```python
from build123d import *

# Parameters (mm, degrees)
BOSS_EXTRUDE1_DEPTH = 8
SKETCH2_R           = 25
BOSS_EXTRUDE2_DEPTH = 1.5
BOSS_EXTRUDE3_START = 1.5
SKETCH3_R           = 25
BOSS_EXTRUDE3_DEPTH = 1.5
SKETCH4_R           = 8
CUT_EXTRUDE1_DEPTH  = 38.027017163
FILLET1_R           = 4


with BuildPart() as part:
    # Sketch1 → Boss-Extrude1 (new body)
    with BuildSketch(Plane(origin=(0, 0, 0), x_dir=(1, 0, 0), z_dir=(0, 1, 0))):
        with BuildLine():
            ThreePointArc((-13.903357517, 20.777310936), (-23.090394822, -9.582988415), (4.894388058, -24.516218418))
            Line((4.894388058, -24.516218418), (1.061192692, -15.28006049))
            Line((1.061192692, -15.28006049), (10.070162151, -11.541153008))
            Line((10.070162151, -11.541153008), (13.903357517, -20.777310936))
            ThreePointArc((13.903357517, -20.777310936), (22.052028681, -11.777437371), (25, 0))
            ThreePointArc((25, 0), (15.85308012, 19.330800571), (-4.894388058, 24.516218418))
            Line((-4.894388058, 24.516218418), (-1.061192692, 15.28006049))
            Line((-1.061192692, 15.28006049), (-10.070162151, 11.541153008))
            Line((-10.070162151, 11.541153008), (-13.903357517, 20.777310936))
        make_face()
    extrude(amount=BOSS_EXTRUDE1_DEPTH)

    # Sketch2 → Boss-Extrude2 (add)
    with BuildSketch(Plane(origin=(0, 8, 0), x_dir=(1, 0, 0), z_dir=(0, 1, 0))):
        with Locations(Location((0, 0, 0), (0, 0, 101.290031001))):
            Circle(SKETCH2_R)
    extrude(amount=BOSS_EXTRUDE2_DEPTH)

    # Sketch3 → Boss-Extrude3 (add)
    with BuildSketch(Plane(origin=(0, 0, 0), x_dir=(-1, 0, 0), z_dir=(0, -1, 0)).offset(BOSS_EXTRUDE3_START)):
        with Locations(Location((0, 0, 0), (0, 0, 90))):
            Circle(SKETCH3_R)
    extrude(amount=-BOSS_EXTRUDE3_DEPTH)

    # Sketch4 → Cut-Extrude1 (cut, through all)
    with BuildSketch(Plane(origin=(0, 9.5, 0), x_dir=(1, 0, 0), z_dir=(0, 1, 0))):
        with Locations(Location((0, 0, 0), (0, 0, 270))):
            Circle(SKETCH4_R)
    extrude(amount=-CUT_EXTRUDE1_DEPTH, mode=Mode.SUBTRACT)

    # Fillet1
    # the kernel refuses this fillet: 4 mm, written as the material it takes off along each edge
    with BuildSketch(Plane(origin=(-13.903357517, 0, -20.777310936), x_dir=(-0.7585073029856567, 0, 0.6516645389442524), z_dir=(0, 1, 0)), Plane(origin=(13.903357517, 0, 20.777310936), x_dir=(0.7585073029856618, 0, -0.6516645389442466), z_dir=(0, 1, 0))) as fillet1_piece_1:
        with BuildLine():
            CenterArc((5.509030911, 3.971210744), FILLET1_R, 161.872235739, 115.006104931)
            Line((1.707570619, 5.215758711), (0, 0))
            ThreePointArc((0, 0), (2.994038539, -0.179932852), (5.988077078, 0))
        make_face()
    extrude(amount=8, mode=Mode.SUBTRACT)


solid = part.part
```
Design review of the part built by this model. Coordinates are the model's own, in mm. A direction names the side the tool comes from. Coordinates: 2 decimals unless noted, no trailing zeros. Order: outer loops, then holes, each group sorted by start corner. A loop starts at its lowest first (then second) coordinate and runs counter-clockwise, first axis right, second up.
1) Mouldability with a two-part tool opening along X and no side actions: class faces 1 (the flat face through (-8, 0, -18)), 2 (the flat face through (6, -1.5, 6)) as +X half, -X half, draft (parallel to the pull), parting line (faces both ways), or undercut.
2) Take a section at A-A, the plane x = 0. Give the boundary of the cut face in (y, z), and give its area (3 significant figures).
3) For faces 3 (the cylindrical face through (14.747, 3.944, 18.105)), 4 (the flat face through (-5.5, 3.94, -13.44)), 5 (the flat face through (-10.923, 3.944, -13.596)), list the 3-axis set-ups (+Z, -Z, +X, -X, +Y, -Y) from which the entire face can be reached by the end or side of a thin tool; tool diameter is ignored.
4) Clearance check with flat-ended pins moving along their axes: pin 1 (6 mm diameter, centred on x = -19, y = 4.5, fed in from +Z); pin 2 (1.5 mm diameter, centred on x = -17, y = 1, fed in from +Z); pin 3 (4 mm diameter, centred on x = 6.5, y = 2.5, fed in from -Z). State where each tip first meets the part, or that it passes through.
5) Take a section at D-D, the plane x = -11. Give the boundary of the cut face in (y, z), and give its area (3 significant figures).
6) Wall thickness on line 1 along Y through (x, z) = (-8.5, -20.5); line 2 along Z through (x, y) = (4, 7.75); line 3 along Z through (x, y) = (-1, 5.5): over which ranges is each line inside the solid? List them lowest first.
7) Take a section at B-B, the plane y = 4.5. Give the boundary of the cut face in (x, z).
8) Take a section at C-C, the plane x = 6.5. Give the boundary of the cut face in (y, z).
Returned:
1. face 1: undercut
1. face 2: draft
2. outline: (-1.5, -25) - (9.5, -25) - (9.5, -8) - (-1.5, -8) - close; (-1.5, 8) - (9.5, 8) - (9.5, 25) - (-1.5, 25) - close
2. area: 374 mm2
3. face 3: +Z
3. face 4: none
3. face 5: -Z
4. pin 1: stops at z = 19.21
4. pin 2: stops at z = 19
4. pin 3: stops at z = -24.59
5. outline: (-1.5, -22.45) - (0, -22.45) - (0, -13.78) - (8, -13.78) - (8, -22.45) - (9.5, -22.45) - (9.5, 22.45) - (-1.5, 22.45) - close
5. area: 425 mm2
6. line 1: y = -1.5 to 0, 8 to 9.5
6. line 2: z = -24.68 to -6.93, 6.93 to 14.06, 22.36 to 24.68
6. line 3: z = -24.98 to -7.94, 7.94 to 24.98
7. outline: (-18.45, -16.88) arc R4 ccw to (-11.8, -15.71) - (-10.07, -11.54) - (-1.06, -15.28) - (-4.89, -24.52) arc R25 ccw to (18.45, 16.88) arc R4 ccw to (11.8, 15.71) - (10.07, 11.54) - (1.06, 15.28) - (4.89, 24.52) arc R25 ccw to start; hole circle Ø16 at (0, 0)
8. outline: (-1.5, -24.14) - (9.5, -24.14) - (9.5, -4.66) - (-1.5, -4.66) - close; (-1.5, 4.66) - (9.5, 4.66) - (9.5, 24.14) - (8, 24.14) - (8, 13.02) - (0, 13.02) - (0, 24.14) - (-1.5, 24.14) - close
